Design review of the part built by this model. Coordinates are the model's own, in mm. A direction names the side the tool comes from. Give positions to 0.01 mm unless a question says otherwise; leave off trailing zeros. Order: outer loops, then holes, each group sorted by start corner. A loop starts at its lowest first (then second) coordinate and runs counter-clockwise, first axis right, second up. Notation, with made-up numbers: (74.25, 18.5) -> (119.25, 18.5) arc R22 ccw to (119.25, 32.5) -> close; hole circle Ø9 at (-17.75, 13.5). An arc over 180 degrees is marked (long way). One line per item, written item: value.
from build123d import *

# Parameters (mm, degrees)
F0_R     = 8.73125
F0_R_2   = 4.7625
F0_R_3   = 3.6068
F1_DEPTH = 1.4986
F2_DEPTH = 2.2606
F3_DEPTH = 5.3848
F4_SIZE  = 0.762
F5_SIZE  = 0.508
F6_SIZE2 = 1.524
F6_SIZE  = 0.1524


with BuildPart() as f1:
    # F0 (on Top) → F1 (new body)
    with BuildSketch(Plane.XY):
        Circle(F0_R)
        Circle(F0_R_2, mode=Mode.SUBTRACT)
        Circle(F0_R_2)
        Circle(F0_R_3, mode=Mode.SUBTRACT)
        Circle(F0_R_3)
    extrude(amount=F1_DEPTH)

    # F0 (on Top) → F2 (join)
    with BuildSketch(Plane.XY):
        Circle(F0_R_2)
        Circle(F0_R_3, mode=Mode.SUBTRACT)
        Circle(F0_R_3)
    extrude(amount=F2_DEPTH)

    # F0 (on Top) → F3 (join)
    with BuildSketch(Plane.XY):
        Circle(F0_R_3)
    extrude(amount=F3_DEPTH)

    # F4
    f4_edges = [f1.edges().sort_by_distance(p)[0] for p in [
        (-8.73125, 0, 1.4986),
    ]]
    chamfer(f4_edges, length=F4_SIZE)

    # F5
    f5_edges = [f1.edges().sort_by_distance(p)[0] for p in [
        (-8.73125, 0, 0),
    ]]
    chamfer(f5_edges, length=F5_SIZE)

    # F6
    f6_edges = [f1.edges().sort_by_distance(p)[0] for p in [
        (-3.6068, 0, 5.3848),
    ]]
    f6_side = f1.faces().sort_by_distance((0, 0, 5.3848))[0]
    chamfer(f6_edges, length=F6_SIZE, length2=F6_SIZE2, reference=f6_side)


solid = f1.part
Item 1: To check wall thickness, follow line 1 along Z through (x, y) = (-3, -3.75); line 2 along X through (y, z) = (1.25, 1.4); line 3 along X through (y, z) = (0, 3.55). State the ranges of each line that lie inside material, in increasing order. Write a range as from..to.
Returned:
line 1: 0..1.5
line 2: -7.97..7.97
line 3: -3.61..3.61
Item 2: Add section C-C on z = 2.5. Give the boundary of the cut face in (x, y).
Returned:
outline: circle Ø7.21 at (0, 0)
Item 3: Add section D-D on z = 4.3. Give the boundary of the cut face in (x, y), plus the area to 3 significant figures.
Returned:
outline: circle Ø7.13 at (0, 0)
area: 39.9 mm²
Item 4: Add section A-A on x = 0. Give the boundary of the cut face in (y, z).
Returned:
outline: (-8.73, 0.51) -> (-8.22, 0) -> (8.22, 0) -> (8.73, 0.51) -> (8.73, 0.74) -> (7.97, 1.5) -> (4.76, 1.5) -> (4.76, 2.26) -> (3.61, 2.26) -> (3.61, 3.86) -> (3.45, 5.38) -> (-3.45, 5.38) -> (-3.61, 3.86) -> (-3.61, 2.26) -> (-4.76, 2.26) -> (-4.76, 1.5) -> (-7.97, 1.5) -> (-8.73, 0.74) -> close
Item 5: Machinability: for faces 1 (the flat face through (0, 0, 5.385)), 2 (the cylindrical face through (-3, -2, 3)), which of the approach directions +Z, -Z, +X, -X, +Y, -Y give a long, thin tool a straight path to every point of the face, cutting with its end or side? Answer none if there is none.
Returned:
face 1: +Z, +X, -X, +Y, -Y
face 2: +Z
